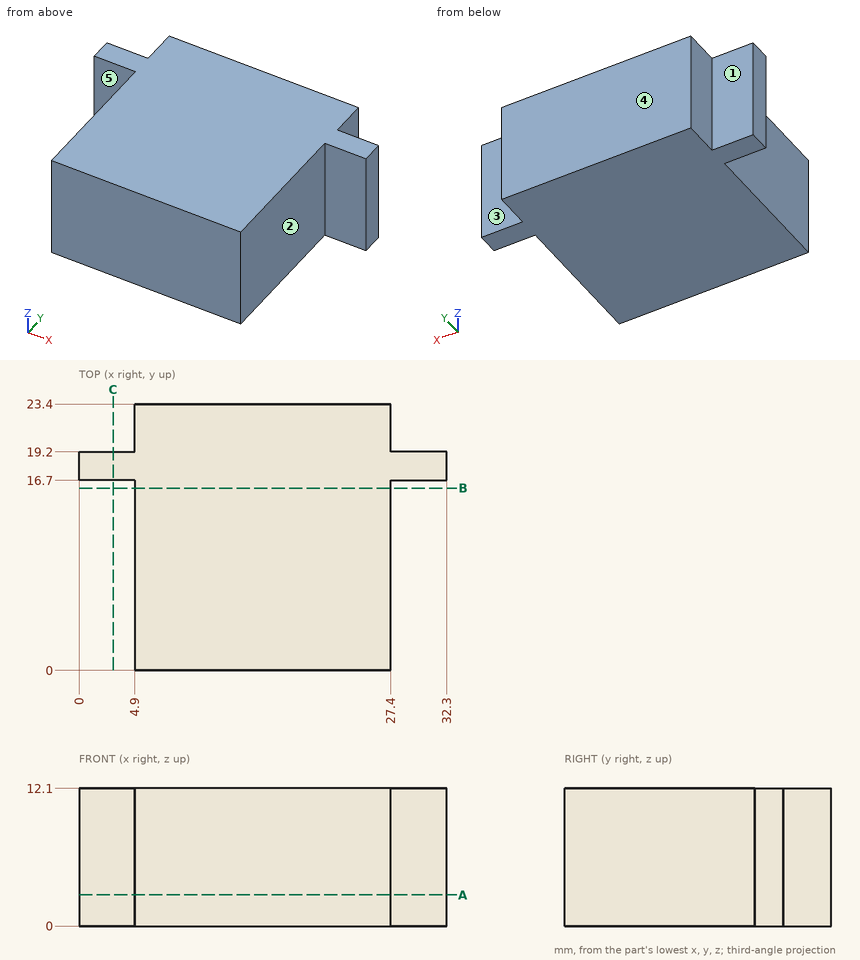
Study the drawing (mm; zero at the part's minimum x, y, z) and answer. A direction names the side the tool comes from. Coordinates: 2 decimals unless noted, no trailing zeros. Loops run counter-clockwise (first coordinate to the right, second up) from the corner with the lowest first, then second, coordinate; pieces in that order, holes last. Notation, with made-up numbers: M 61.25,35.25 L 112.25,35.25 A38 ccw 112.25,74.25 Z; hole C 79.25,62 d2. An arc over 180 degrees is marked long. Answer as a JSON object with one key per item and string values. Group by question number.
Item 1: Each of these flat-tipped pins is pushed along its axis until it touches: P1, Ø1.3, axis at y = 21.5, z = 7.5, coming from the -X side; P2, Ø2.5, axis at x = 29.5, z = 7.5, coming from the +Y side; P3, Ø2, axis at x = 16, z = 8.5, coming from the -Y side; P4, Ø2, axis at y = 21, z = 4.5, coming from the +X side. Where does it stop, or does it pass through?
Item 2: Which of the six approach directions +Z, -Z, +X, -X, +Y, -Y give full straight-line access (tool end or side, diameter ignored) to the marked faces 1, 2, 3, 4 and 5?
Item 3: Section C-C (x = 3) is taken. Write down the section's boundary in (y, z), and give its area (4 significant figures).
Item 4: Consider L1, parallel to X at y = 6.5, z = 2; L2, parallel to Y at x = 4, z = 3.75. Determine where each line is inside the solid, lowest interval first.
Item 5: Section B-B (y = 16) is taken. Write down the section's boundary in (x, z), and give its area (3 significant figures).
Item 6: Section A-A (z = 2.75) is taken. Write down the section's boundary in (x, y), and give its area (3 significant figures).
Solved:
{
 "1": {"P1": "stops at x = 4.9", "P2": "stops at y = 19.2", "P3": "stops at y = 0", "P4": "stops at x = 27.4"},
 "2": {"face 1": "+Z, -Z, -X, +Y", "face 2": "+Z, -Z, +X, -Y", "face 3": "+Z, -Z, +X, +Y", "face 4": "+Z, -Z, +X, -X, +Y", "face 5": "+Z, -Z, -X, -Y"},
 "3": {"outline": "M 16.7,0 L 19.2,0 L 19.2,12.1 L 16.7,12.1 Z", "area": "30.25 mm2"},
 "4": {"L1": "x = 4.9 to 27.4", "L2": "y = 16.7 to 19.2"},
 "5": {"outline": "M 4.9,0 L 27.4,0 L 27.4,12.1 L 4.9,12.1 Z", "area": "272 mm2"},
 "6": {"outline": "M 0,16.7 L 4.9,16.7 L 4.9,0 L 27.4,0 L 27.4,16.7 L 32.3,16.7 L 32.3,19.2 L 27.4,19.2 L 27.4,23.4 L 4.9,23.4 L 4.9,19.2 L 0,19.2 Z", "area": "551 mm2"}
}
